Design review of the part built by this model. Coordinates are the model's own, in mm. A direction names the side the tool comes from. Coordinates: 2 decimals unless noted, no trailing zeros. Write each loop counter-clockwise with the first axis right and the second up, starting at its lowest first coordinate (ties: lowest second). Pieces come first, ordered by that corner, then holes. Notation, with made-up numbers: (79.5, 13) -> (112.5, 13) arc R27 cw to (112.5, 39) -> close; hole circle Ø9 at (-23.75, -37.5). An arc over 180 degrees is marked (long way). One line per question, with ' | ' between items. Start each with the question number.
Q1. Add section B-B on x = -7.5. State the section outline as (y, z) points, and give its area (3 significant figures).
Q2. Add section A-A on z = 0.5. State the section outline as (x, y) points, and give its area (3 significant figures).
Q3. For faces 1 (the flat face through (0, -2, 10)), 2 (the cylindrical face through (-0.97, 5.54, -1.27)), 3 (the flat face through (-7, -7, 11)), 4 (the flat face through (0.029, -6.314, 17.57)), list the 3-axis set-ups (+Z, -Z, +X, -X, +Y, -Y) from which the entire face can be reached by the end or side of a thin tool; tool diameter is ignored.
Q4. Add section D-D on y = 2.5. State the section outline as (x, z) points, and give its area (3 significant figures).
Q5. Add section C-C on y = 5. State the section outline as (x, z) points.
Q6. Wall thickness on probe 1 along X at (y, z) = (5.5, 0); probe 2 along Y at (x, z) = (-9, 9); probe 3 along X at (y, z) = (5.7, 0): over which ranges is each line inside the solid? List them lowest first.
Q7. For P1, Ø10, axis at x = -7.5, y = -6.5, coming from the -Z side; P2, Ø1.9, axis at x = 0, z = 0, coming from the +Y side; P3, Ø1.5, axis at x = -6, y = 3.5, coming from the +Z side; P4, Ø2.5, axis at y = 5, z = 6, coming from the +X side, all flat-tipped, find the tip position at first contact; note any pin that passes through.
Q8. Draft analysis for pull direction X (two halves, no side actions). For faces 5 (the flat face through (10, 5, 5)), 6 (the cylindrical face through (-0.785, -11.046, 20.218)), 7 (the flat face through (-2.4, 0.3, 15)), 8 (the cylindrical face through (-14, 6, 0)), state which applies: pulls with the +X half, pulls with the -X half, needs draft (parallel to the pull), parting line crosses it, or undercut.
from build123d import *

# Parameters (mm, degrees)
SKETCH_1_W          = 20
SKETCH_1_H          = 20
EXTRUDE_1_DEPTH     = 8
SKETCH_2_R          = 4
EXTRUDE_2_DEPTH     = 25
SKETCH_3_R          = 4
EXTRUDE_3_DEPTH     = 25
SKETCH_4_R          = 1.6
CUT_EXTRUDE_1_DEPTH = 46.952030516
EXTRUDE_4_DEPTH     = 15
CUT_EXTRUDE_START   = -10
CUT_EXTRUDE_5_DEPTH = 10
SKETCH_11_R         = 2.05
CUT_EXTRUDE_6_DEPTH = 10
SKETCH_12_R         = 2.05
CUT_EXTRUDE_7_DEPTH = 10
FILLET_3_R          = 5


with BuildPart() as part:
    # 草圖1 → 填料-伸長1 (new body)
    with BuildSketch(Plane(origin=(0, 0, 0), x_dir=(1, 0, 0), z_dir=(0, 1, 0))):
        Rectangle(SKETCH_1_W, SKETCH_1_H)
    extrude(amount=EXTRUDE_1_DEPTH)

    # 草圖2 → 填料-伸長2 (add)
    with BuildSketch(Plane(origin=(0, -1.618631476, 1.929009876), x_dir=(1, 0, 0), z_dir=(0, -0.6427876096865406, 0.7660444431189771))):
        with Locations((0, 6.427876097)):
            Circle(SKETCH_2_R)
    extrude(amount=EXTRUDE_2_DEPTH)

    # 草圖3 → 填料-伸長3 (add)
    with BuildSketch(Plane(origin=(-1.929009876, -1.618631476, 0), x_dir=(0, 0, 1), z_dir=(-0.7660444431189771, -0.6427876096865406, 0))):
        with Locations((0, 6.427876097)):
            Circle(SKETCH_3_R)
    extrude(amount=EXTRUDE_3_DEPTH)

    # 草圖4 → 除料-伸長1 (cut, through all)
    with BuildSketch(Plane(origin=(0, 8, 0), x_dir=(1, 0, 0), z_dir=(0, 1, 0))):
        with Locations(Location((0, 0, 0), (0, 0, 270))):
            Circle(SKETCH_4_R)
        with BuildLine():
            Line((0, 10), (10, 10))
            Line((10, 10), (10, 0))
            ThreePointArc((10, 0), (7.071067812, 7.071067812), (0, 10))
        make_face()
    extrude(amount=-CUT_EXTRUDE_1_DEPTH, mode=Mode.SUBTRACT)

    # 草圖9 → 填料-伸長4 (add)
    with BuildSketch(Plane(origin=(0, 8, 0), x_dir=(1, 0, 0), z_dir=(0, 1, 0))):
        Polygon((-10, 10), (-15, 10), (-15, -15), (10.028553892, -15), (10, -10), (-10, -10), align=None)
    extrude(amount=-EXTRUDE_4_DEPTH)

    # 草圖10 → 除料-伸長5 (cut)
    with BuildSketch(Plane.XZ.offset(7).offset(CUT_EXTRUDE_START)):
        with BuildLine():
            Line((10, 0), (10, 10))
            Line((10, 10), (-10, 10))
            Line((-10, 10), (-10, -10))
            Line((-10, -10), (0, -10))
            ThreePointArc((0, -10), (7.071067812, -7.071067812), (10, 0))
        make_face()
    extrude(amount=CUT_EXTRUDE_5_DEPTH, mode=Mode.SUBTRACT)

    # 草圖11 → 除料-伸長6 (cut)
    with BuildSketch(Plane(origin=(-21.080120954, -17.688321718, 0), x_dir=(0, 0, 1), z_dir=(-0.7660444431189772, -0.6427876096865405, 0))):
        with Locations(Location((0, 6.427876097, 0), (0, 0, 270))):
            Circle(SKETCH_11_R)
    extrude(amount=-CUT_EXTRUDE_6_DEPTH, mode=Mode.SUBTRACT)

    # 草圖12 → 除料-伸長7 (cut)
    with BuildSketch(Plane(origin=(0, -17.688321718, 21.080120954), x_dir=(1, 0, 0), z_dir=(0, -0.6427876096865405, 0.7660444431189771))):
        with Locations(Location((0, 6.427876097, 0), (0, 0, 270))):
            Circle(SKETCH_12_R)
    extrude(amount=-CUT_EXTRUDE_7_DEPTH, mode=Mode.SUBTRACT)

    # 圓角3
    fillet_3_edges = [part.edges().sort_by_distance(p)[0] for p in [
        (-2.485723054, 8, 15),
        (-15, 8, 2.5),
        (-15, 0.5, 15),
    ]]
    fillet(fillet_3_edges, radius=FILLET_3_R)


solid = part.part
Output values:
1) outline: (-7, 10) -> (3, 10) -> (3, -10) -> (8, -10) -> (8, 10) arc R5 ccw to (3, 15) -> (-7, 15) -> close | area: 170 mm2
2) outline: (-27.76, -9.72) -> (-26.49, -11.24) -> (-18.83, -4.81) -> (-16.27, -7.86) -> (-23.93, -14.29) -> (-22.66, -15.8) -> (-12.17, -7) -> (-10, -7) -> (-10, 3) -> (-1.52, 3) -> (-1.52, 8) -> (-10, 8) arc R5 ccw to (-15, 3) -> (-15, 0.99) -> close; (1.52, 3) -> (10, 3) -> (10, 8) -> (1.52, 8) -> close | area: 224 mm2
3) face 1: -Z, +X, -Y | face 2: +Y, -Y | face 3: -Y | face 4: none
4) outline: (-15, -10) -> (-10, -10) -> (-10, 10) -> (10, 10) -> (10.03, 15) -> (-10, 15) arc R5 ccw to (-15, 10) -> close | area: 220 mm2
5) outline: (-14.58, -10) -> (0, -10) arc R10 ccw to (10, 0) -> (10, 10) -> (10.03, 14.58) -> (-10, 14.58) arc R4.58 ccw to (-14.58, 10) -> close; hole circle Ø3.2 at (0, 0)
6) probe 1: x = -14.33 to -1.6, 1.6 to 10 | probe 2: y = 3 to 8 | probe 3: x = -14.21 to -1.6, 1.6 to 10
7) P1: stops at z = -10 | P2: passes through | P3: stops at z = 15 | P4: stops at x = 10
8) face 5: pulls with the +X half | face 6: undercut | face 7: needs draft | face 8: pulls with the -X half
